from build123d import *

# Parameters (mm, degrees)
F0_W     = 203.2
F0_H     = 127
F1_DEPTH = 127
F3_DEPTH = 76.2
F4_SIZE2 = 101.6
F4_SIZE  = 76.2
F5_R     = 5.08
F6_R     = 15.24
F7_DEPTH = 76.2


with BuildPart() as f1:
    # F0 (on Front) → F1 (new body)
    with BuildSketch(Plane.XZ):
        Rectangle(F0_W, F0_H)
    extrude(amount=F1_DEPTH)

    # F2 (on face) → F3 (cut)
    with BuildSketch(Plane.XZ.offset(127)):
        Polygon((101.6, 63.5), (0, 63.5), (0, 0), (-39.1343943775, 0), (-39.1343943775, -63.5), (101.6, -63.5), align=None)
    extrude(amount=-F3_DEPTH, mode=Mode.SUBTRACT)

    # F4
    f4_edges = [f1.edges().sort_by_distance(p)[0] for p in [
        (101.6, -25.4, 63.5),
    ]]
    f4_side = f1.faces().sort_by_distance((-21.771429, -52.614286, 63.5))[0]
    chamfer(f4_edges, length=F4_SIZE, length2=F4_SIZE2, reference=f4_side)

    # F5
    f5_edges = [f1.edges().sort_by_distance(p)[0] for p in [
        (-38.1, 0, 63.5),
        (25.4, -25.4, 63.5),
        (-101.6, -63.5, 63.5),
        (12.7, -50.8, 63.5),
        (-50.8, -127, 63.5),
        (0, -88.9, 63.5),
        (0, -127, 31.75),
        (-19.567197, -127, 0),
        (-39.134394, -127, -31.75),
        (-70.367197, -127, -63.5),
        (-101.6, -127, 0),
        (-39.134394, -88.9, 0),
        (-39.134394, -88.9, -63.5),
        (-39.134394, -50.8, -31.75),
        (0, -88.9, 0),
        (0, -50.8, 31.75),
        (63.5, -50.8, 12.7),
        (101.6, -50.8, -50.8),
        (-19.567197, -50.8, 0),
        (31.232803, -50.8, -63.5),
        (63.5, 0, 12.7),
        (101.6, -25.4, -38.1),
        (101.6, 0, -50.8),
        (101.6, -25.4, -63.5),
        (-101.6, 0, 0),
        (0, 0, -63.5),
        (-101.6, -63.5, -63.5),
    ]]
    fillet(f5_edges, radius=F5_R)

    # F6 (on face) → F7 (cut)
    with BuildSketch(Plane.XZ.offset(50.8)):
        with Locations((12.1788298711, -30.0629306585)):
            Circle(F6_R)
    extrude(amount=-F7_DEPTH, mode=Mode.SUBTRACT)


solid = f1.part
Work out the finished part from the listing and answer in its coordinate system (mm). A direction names the side the tool comes from. Round coordinates to 2 decimals unless told otherwise and drop trailing zeros. Write each loop counter-clockwise with the first axis right and the second up, starting at its lowest first coordinate (ties: lowest second). Pieces come first, ordered by that corner, then holes. Notation, with made-up numbers: (70, 74) -> (109, 74) arc R22 cw to (109, 105) -> close; hole circle Ø8 at (86.5, 25). An arc over 180 degrees is marked (long way). Answer as CSV lines item,"result". Start each with the question number.
(1) The mould has two halves that part along Y. Classify faces 1 (the cylindrical face through (-50.16, -125.472, 62.051)), 2 (the cylindrical face through (100.151, -25.684, -61.972)), 3 (the cylindrical face through (1.351, -1.449, -61.972)): +Y half, -Y half, draft (parallel to the pull), parting line (faces both ways), or undercut.
(2) The part is cut by section B-B, the plane y = -116. Give the vertices of the cut face in (x, z).
(3) Find the intervals of material crossed by probe 1 along Y at (x, z) = (-15, -18); probe 2 along X at (y, z) = (-21.5, -24) (3 decimals); probe 3 along X at (y, z) = (-119.5, 51), in increasing order.
(4) The part is cut by section C-C, the plane y = -18.5. Give the vertices of the cut face in (x, z).
(5) A tool of negligible diameter and unlimited length cuts with its end or side. For faces 4 (the flat face through (30, -50.8, -12)), 5 (the cylindrical face through (1.528, -52.249, 31.377)), from which of +Z, -Z, +X, -X, +Y, -Y can it reach the whole face along a straight path? Write none if from no direction.
(6) The part is cut by section A-A, the plane x = 12. Give the vertices of the cut face in (y, z), then the cut area to 3 significant figures.
(7) Each of these flat-tipped pins is pushed along its axis until it touches: pin 1 (23 mm diameter, centred on x = -16.5, y = -80, fed in from -Z); pin 2 (12 mm diameter, centred on x = 38, z = 4.5, fed in from +Y); pin 3 (6 mm diameter, centred on x = -32, y = -51, fed in from -Z). Where does it stop, or does it pass through?
Output values:
1,face 1,"-Y half"
1,face 2,"draft"
1,face 3,"+Y half"
2,outline,"(-101.6, -58.42) arc R5.08 ccw to (-96.52, -63.5) -> (-44.21, -63.5) arc R5.08 ccw to (-39.13, -58.42) -> (-39.13, -5.08) arc R5.08 cw to (-34.05, 0) -> (-5.08, 0) arc R5.08 ccw to (0, 5.08) -> (0, 58.42) arc R5.08 ccw to (-5.08, 63.5) -> (-96.52, 63.5) arc R5.08 ccw to (-101.6, 58.42) -> close"
3,probe 1,"y = -50.8 to 0"
3,probe 2,"x = -101.6 to -1.803, 26.161 to 91.025"
3,probe 3,"x = -101.6 to 0"
4,outline,"(-101.6, -58.42) arc R5.08 ccw to (-96.52, -63.5) -> (96.52, -63.5) arc R5.08 ccw to (101.6, -58.42) -> (101.6, -39.79) arc R5.08 ccw to (100.58, -36.75) -> (26.92, 61.47) arc R5.08 ccw to (22.86, 63.5) -> (-96.52, 63.5) arc R5.08 ccw to (-101.6, 58.42) -> close; hole circle Ø30.48 at (12.18, -30.06)"
5,face 4,"-Z, +X, -Y"
5,face 5,"+Z, -Z, +X, -Y"
6,outline,"(-50.8, -58.42) arc R5.08 ccw to (-45.72, -63.5) -> (-5.08, -63.5) arc R5.08 ccw to (0, -58.42) -> (0, -45.3) -> (-50.8, -45.3) -> close; (-50.8, -14.82) -> (0, -14.82) -> (0, 58.42) arc R5.08 ccw to (-5.08, 63.5) -> (-45.72, 63.5) arc R5.08 ccw to (-50.8, 58.42) -> close"
6,area,"4,880 mm²"
7,pin 1,"stops at z = 0"
7,pin 2,"stops at y = 0"
7,pin 3,"stops at z = -62.96"
